Work out the finished part from the listing and answer in its coordinate system (mm). A direction names the side the tool comes from. Round coordinates to 2 decimals unless told otherwise and drop trailing zeros. Write each loop counter-clockwise with the first axis right and the second up, starting at its lowest first coordinate (ties: lowest second). Pieces come first, ordered by that corner, then holes. Notation, with made-up numbers: M 19,-4 L 60,-4 A13 ccw 60,18 Z; hole C 47.25,21.25 d3. An arc over 180 degrees is marked long. One line per item, written item: value. Start each with the question number.
Q1. Find section C-C (z = 15.5). Count the separate pieces of the cut face and the enclosed holes in it, and give its area (3 significant figures).
Q2. Given pin 1 Ø4 at (x, z) = (40, -22) entering from +Y; pin 2 Ø0.6 at (x, y) = (47, 1) entering from -Z; pin 3 Ø4 at (x, z) = (-36.5, 15.5) entering from -Y; pin 4 Ø6 at (x, z) = (40, 22) entering from -Y, each flat-ended and moving along its own axis, determine where each tip first touches the part or whether it passes through.
Q3. The mould has two halves that part along X. Classify faces 4 (the flat face through (-43.92, 7.8, -25.8)), 5 (the cylindrical face through (-40.488, 2.022, -19.804)), 6 (the flat face through (44, 4, 26)): released by +X, released by -X, zero draft, split by the parting line, or undercut.
Q4. Find section B-B (x = -21). Write down the section's boundary in (y, z).
Q5. Find section A-A (z = 0). Write down the section's boundary in (x, y).
Q6. Consider probe 1 along Z at (x, y) = (-40, 1.15); probe 2 along X at (y, z) = (4.9, 15.5); probe 3 along Z at (x, y) = (41, 7.5). Determine where each line is inside the solid, lowest interval first.
Q7. A tool of negligible diameter and unlimited length cuts with its end or side. For faces 1 (the flat face through (-44, 4, -26)), 2 (the flat face through (-42.28, 7.8, 19.1)), 3 (the flat face through (21, 7, 0)), from which of +Z, -Z, +X, -X, +Y, -Y can it reach the whole face along a straight path? Write none if from no direction.
from build123d import *

# Parameters (mm, degrees)
SKETCH1_W                        = 96
SKETCH1_H                        = 60
BOSS_EXTRUDE1_DEPTH              = 8
CHAMFER1_SIZE                    = 8
HOLE2_D                          = 16
SKETCH6_R                        = 8
CUT_EXTRUDE1_DEPTH               = 7
CBORE_FOR_M3_SHCS1_OUTLINE_R     = 3.25
CBORE_FOR_M3_SHCS1_DEPTH         = 3.2
CBORE_START                      = 3.2
CBORE_FOR_M3_SHCS1_2_OUTLINE_R   = 1.7
CBORE_FOR_M3_SHCS1_2_DEPTH       = 4.8
CHAMFER3_SIZE                    = 0.4
SKETCH10_R                       = 3
SKETCH10_R_2                     = 2.25
BOSS_EXTRUDE2_DEPTH              = 2
CHAMFER4_SIZE                    = 0.2
CHAMFER4_OF_SKETCH_PATTERN1_SIZE = 0.2
CUT_EXTRUDE2_DEPTH               = 4
SKETCH14_R                       = 4.025
SKETCH14_R_2                     = 2.25
BOSS_EXTRUDE3_DEPTH              = 4.2
CUT_EXTRUDE3_DEPTH               = 4.4
CHAMFER6_SIZE                    = 0.4
CHAMFER7_SIZE                    = 0.4
CUT_EXTRUDE4_DEPTH               = 1
CHAMFER8_SIZE                    = 0.2


# Read off the part's stored shape, not the designer's step: CBORE for M4 SHCS1, CBORE for M3 SHCS1
with BuildPart() as part:
    # Sketch1 → Boss-Extrude1 (new body)
    with BuildSketch(Plane(origin=(0, 0, 0), x_dir=(1, 0, 0), z_dir=(0, 1, 0))):
        Rectangle(SKETCH1_W, SKETCH1_H)
    extrude(amount=BOSS_EXTRUDE1_DEPTH)

    # CBORE for M4 SHCS1 outline → CBORE for M4 SHCS1 (revolve, cut)
    with BuildSketch(Plane(origin=(40, 0, 22), x_dir=(1, 0, 0), z_dir=(0, 0, 1))):
        Polygon((0, 0), (2.25, 0), (2.25, 3.8), (4, 3.8), (4, 7.975), (4.025, 8), (0, 8), align=None)
    revolve(axis=Axis((40, 0, 22), (0, 1, 0)), mode=Mode.SUBTRACT)

    # CBORE for M4 SHCS1 2 outline → CBORE for M4 SHCS1 2 (revolve, cut)
    with BuildSketch(Plane(origin=(-40, 0, -22), x_dir=(1, 0, 0), z_dir=(0, 0, 1))):
        Polygon((0, 8), (0, 0), (2.25, 0), (2.25, 3.8), (4, 3.8), (4, 7.975), (4.025, 8), align=None)
    revolve(axis=Axis((-40, 0, -22), (0, 1, 0)), mode=Mode.SUBTRACT)

    # CBORE for M4 SHCS1 3 outline → CBORE for M4 SHCS1 3 (revolve, cut)
    with BuildSketch(Plane(origin=(-40, 0, 22), x_dir=(1, 0, 0), z_dir=(0, 0, 1))):
        Polygon((0, 8), (0, 0), (2.25, 0), (2.25, 3.8), (4, 3.8), (4, 7.975), (4.025, 8), align=None)
    revolve(axis=Axis((-40, 0, 22), (0, 1, 0)), mode=Mode.SUBTRACT)

    # CBORE for M4 SHCS1 4 outline → CBORE for M4 SHCS1 4 (revolve, cut)
    with BuildSketch(Plane(origin=(40, 0, -22), x_dir=(1, 0, 0), z_dir=(0, 0, 1))):
        Polygon((0, 8), (0, 0), (2.25, 0), (2.25, 3.8), (4, 3.8), (4, 7.975), (4.025, 8), align=None)
    revolve(axis=Axis((40, 0, -22), (0, 1, 0)), mode=Mode.SUBTRACT)

    # Chamfer1
    chamfer1_edges = [part.edges().sort_by_distance(p)[0] for p in [
        (48, 4, 30),
        (-48, 4, 30),
        (-48, 4, -30),
        (48, 4, -30),
    ]]
    chamfer(chamfer1_edges, length=CHAMFER1_SIZE)

    # Hole2 (through all)
    with Locations(Plane(origin=(0, 8, 0), x_dir=(1, 0, 0), z_dir=(0, 1, 0))):
        with Locations((-21, 0)):
            Hole(HOLE2_D / 2)

    # Sketch6 → Cut-Extrude1 (cut)
    with BuildSketch(Plane.XZ):
        with Locations(Location((21, 0, 0), (0, 0, 270))):
            Circle(SKETCH6_R)
    extrude(amount=-CUT_EXTRUDE1_DEPTH, mode=Mode.SUBTRACT)

    # CBORE for M3 SHCS1 outline → CBORE for M3 SHCS1 (cut)
    with BuildSketch(Plane(origin=(0, 0, 0), x_dir=(1, 0, 0), z_dir=(0, 1, 0))):
        with Locations((-5.5, 15.5)):
            Circle(CBORE_FOR_M3_SHCS1_OUTLINE_R)
        with Locations((-36.5, 15.5)):
            Circle(CBORE_FOR_M3_SHCS1_OUTLINE_R)
        with Locations((-36.5, -15.5)):
            Circle(CBORE_FOR_M3_SHCS1_OUTLINE_R)
        with Locations((-5.5, -15.5)):
            Circle(CBORE_FOR_M3_SHCS1_OUTLINE_R)
    extrude(amount=CBORE_FOR_M3_SHCS1_DEPTH, mode=Mode.SUBTRACT)

    # CBORE for M3 SHCS1 2 outline → CBORE for M3 SHCS1 2 (cut)
    with BuildSketch(Plane(origin=(0, 0, 0), x_dir=(1, 0, 0), z_dir=(0, 1, 0)).offset(CBORE_START)):
        with Locations((-5.5, 15.5)):
            Circle(CBORE_FOR_M3_SHCS1_2_OUTLINE_R)
        with Locations((-36.5, 15.5)):
            Circle(CBORE_FOR_M3_SHCS1_2_OUTLINE_R)
        with Locations((-36.5, -15.5)):
            Circle(CBORE_FOR_M3_SHCS1_2_OUTLINE_R)
        with Locations((-5.5, -15.5)):
            Circle(CBORE_FOR_M3_SHCS1_2_OUTLINE_R)
    extrude(amount=CBORE_FOR_M3_SHCS1_2_DEPTH, mode=Mode.SUBTRACT)

    # Chamfer3
    chamfer3_edges = [part.edges().sort_by_distance(p)[0] for p in [
        (-39.75, 0, 15.5),
        (-8.75, 0, 15.5),
        (37.75, 0, 22),
        (-42.25, 0, -22),
        (-42.25, 0, 22),
        (37.75, 0, -22),
        (-13, 0, 0),
        (-8.75, 0, -15.5),
        (-39.75, 0, -15.5),
    ]]
    chamfer(chamfer3_edges, length=CHAMFER3_SIZE)

    # Sketch10 → Boss-Extrude2 (add)
    with BuildSketch(Plane.XZ):
        with Locations(Location((-40, 22, 0), (0, 0, 270))):
            Circle(SKETCH10_R)
        with Locations(Location((-40, 22, 0), (0, 0, 90))):
            Circle(SKETCH10_R_2, mode=Mode.SUBTRACT)
    boss_extrude2 = extrude(amount=BOSS_EXTRUDE2_DEPTH)

    # Chamfer4
    chamfer4_edges = [part.edges().sort_by_distance(p)[0] for p in [
        (-40, -2, 25),
    ]]
    chamfer(chamfer4_edges, length=CHAMFER4_SIZE)

    # Sketch-Pattern1: Boss-Extrude2 at 3 more places
    with Locations((80, 0, 0), (80, 0, -44), (0, 0, -44)):
        add(boss_extrude2)

    # Chamfer4 of Sketch-Pattern1
    chamfer4_of_sketch_pattern1_edges = [part.edges().sort_by_distance(p)[0] for p in [
        (40, -2, 25),
        (40, -2, -19),
        (-40, -2, -19),
    ]]
    chamfer(chamfer4_of_sketch_pattern1_edges, length=CHAMFER4_OF_SKETCH_PATTERN1_SIZE)

    # Sketch13 → Cut-Extrude2 (cut, symmetric)
    with BuildSketch(Plane.XY):
        Polygon((-48, 0), (-46, 0), (-48, 1.154700538), align=None)
    cut_extrude2 = extrude(amount=CUT_EXTRUDE2_DEPTH, both=True, mode=Mode.SUBTRACT)

    # Mirror1: Cut-Extrude2 across plane
    add(cut_extrude2.mirror(Plane(origin=(0, 0, 0), x_dir=(0, 0, 1), z_dir=(1, 0, 0))), mode=Mode.SUBTRACT)

    # Sketch14 → Boss-Extrude3 (add)
    # profile 1 of 4: a face of its own
    with BuildSketch(Plane(origin=(0, 8, 0), x_dir=(1, 0, 0), z_dir=(0, 1, 0))):
        with Locations((40, 22)):
            Circle(SKETCH14_R)
        with Locations(Location((40, 22, 0), (0, 0, 270))):
            Circle(SKETCH14_R_2, mode=Mode.SUBTRACT)
    # profile 2 of 4: a face of its own
    with BuildSketch(Plane(origin=(0, 8, 0), x_dir=(1, 0, 0), z_dir=(0, 1, 0))):
        with Locations((-40, -22)):
            Circle(SKETCH14_R)
        with Locations(Location((-40, -22, 0), (0, 0, 270))):
            Circle(SKETCH14_R_2, mode=Mode.SUBTRACT)
    # profile 3 of 4: a face of its own
    with BuildSketch(Plane(origin=(0, 8, 0), x_dir=(1, 0, 0), z_dir=(0, 1, 0))):
        with Locations((-40, 22)):
            Circle(SKETCH14_R)
        with Locations(Location((-40, 22, 0), (0, 0, 270))):
            Circle(SKETCH14_R_2, mode=Mode.SUBTRACT)
    # profile 4 of 4: a face of its own
    with BuildSketch(Plane(origin=(0, 8, 0), x_dir=(1, 0, 0), z_dir=(0, 1, 0))):
        with Locations((40, -22)):
            Circle(SKETCH14_R)
        with Locations(Location((40, -22, 0), (0, 0, 270))):
            Circle(SKETCH14_R_2, mode=Mode.SUBTRACT)
    extrude(amount=-BOSS_EXTRUDE3_DEPTH)

    # Sketch15 → Cut-Extrude3 (cut)
    with BuildSketch(Plane(origin=(0, 8, 0), x_dir=(1, 0, 0), z_dir=(0, 1, 0))):
        Polygon((-40, 25.983716857), (-43.45, 23.991858429), (-43.45, 20.008141571), (-40, 18.016283143), (-36.55, 20.008141571), (-36.55, 23.991858429), align=None)
    cut_extrude3 = extrude(amount=-CUT_EXTRUDE3_DEPTH, mode=Mode.SUBTRACT)

    # Sketch-Pattern2: Cut-Extrude3 at 3 more places
    with Locations((0, 0, 44), (80, 0, 44), (80, 0, 0)):
        add(cut_extrude3, mode=Mode.SUBTRACT)

    # Chamfer6
    chamfer6_edges = [part.edges().sort_by_distance(p)[0] for p in [
        (-38.2, 8, 15.5),
        (-7.2, 8, 15.5),
        (-38.275, 8, -24.987787643),
        (-41.725, 8, -24.987787643),
        (-43.45, 8, -22),
        (-41.725, 8, -19.012212357),
        (-38.275, 8, -19.012212357),
        (-36.55, 8, -22),
        (41.725, 8, -24.987787643),
        (38.275, 8, -24.987787643),
        (36.55, 8, -22),
        (38.275, 8, -19.012212357),
        (41.725, 8, -19.012212357),
        (43.45, 8, -22),
        (41.725, 8, 19.012212357),
        (38.275, 8, 19.012212357),
        (36.55, 8, 22),
        (38.275, 8, 24.987787643),
        (41.725, 8, 24.987787643),
        (43.45, 8, 22),
        (-38.275, 8, 19.012212357),
        (-41.725, 8, 19.012212357),
        (-43.45, 8, 22),
        (-41.725, 8, 24.987787643),
        (-38.275, 8, 24.987787643),
        (-36.55, 8, 22),
        (48, 8, 0),
        (0, 8, 30),
        (0, 8, -30),
        (-48, 8, 0),
        (-44, 8, 26),
        (-44, 8, -26),
        (44, 8, -26),
        (44, 8, 26),
        (-13, 8, 0),
        (-7.2, 8, -15.5),
        (-38.2, 8, -15.5),
    ]]
    chamfer(chamfer6_edges, length=CHAMFER6_SIZE)

    # Chamfer7
    chamfer7_edges = [part.edges().sort_by_distance(p)[0] for p in [
        (21, 0, 8),
        (21, 7, 8),
    ]]
    chamfer(chamfer7_edges, length=CHAMFER7_SIZE)

    # Sketch16 → Cut-Extrude4 (cut)
    with BuildSketch(Plane(origin=(0, 8, 0), x_dir=(1, 0, 0), z_dir=(0, 1, 0))):
        Polygon((-42.1, 17.1), (-38.1, 21.1), (-3.9, 21.1), (0.1, 17.1), (0.1, -17.1), (-3.9, -21.1), (-38.1, -21.1), (-42.1, -17.1), align=None)
    extrude(amount=-CUT_EXTRUDE4_DEPTH, mode=Mode.SUBTRACT)

    # Chamfer8
    chamfer8_edges = [part.edges().sort_by_distance(p)[0] for p in [
        (-20.025, 8, -21.1),
        (-41.57163337, 8, -17.62836663),
        (-42.1, 8, 0),
        (-41.57163337, 8, 17.62836663),
        (-20.025, 8, 21.1),
        (-1.9, 8, 19.1),
        (0.1, 8, 0),
        (-1.9, 8, -19.1),
    ]]
    chamfer(chamfer8_edges, length=CHAMFER8_SIZE)


solid = part.part
The answers:
1. separate pieces: 3
1. enclosed holes: 0
1. area: 658 mm2
2. pin 1: through
2. pin 2: z = -23.3
2. pin 3: y = 3.2
2. pin 4: y = -2
3. face 4: released by -X
3. face 5: undercut
3. face 6: released by +X
4. outline: M 0,-30 L 7.6,-30 L 8,-29.6 L 8,-21.3 L 7.8,-21.1 L 7,-21.1 L 7,-8 L 0.4,-8 L 0,-8.4 Z; M 0,8.4 L 0.4,8 L 7,8 L 7,21.1 L 7.8,21.1 L 8,21.3 L 8,29.6 L 7.6,30 L 0,30 Z
5. outline: M -48,1.15 L -46,0 L -29.4,0 L -29,0.4 L -29,7 L -42.1,7 L -42.1,7.8 L -42.3,8 L -47.6,8 L -48,7.6 Z; M -13,0.4 L -12.6,0 L 12.6,0 L 13,0.4 L 13,6.6 L 13.4,7 L 28.6,7 L 29,6.6 L 29,0.4 L 29.4,0 L 46,0 L 48,1.15 L 48,7.6 L 47.6,8 L 0.3,8 L 0.1,7.8 L 0.1,7 L -13,7 Z
6. probe 1: -30 to -24.25, -19.75 to 19.75, 24.25 to 30
6. probe 2: -48 to -38.2, -34.8 to -7.2, -3.8 to 48
6. probe 3: -29 to -25.41, -18.59 to 18.59, 25.41 to 29
7. face 1: -Z, -X, +Y, -Y
7. face 2: +Y
7. face 3: -Y
